The listing builds one solid part. Answer for the finished solid, in the listing's coordinates (mm). Face numbers are marked on the shaded views. Coordinates: 2 decimals unless noted, no trailing zeros. Order: outer loops, then holes, each group sorted by start corner. A loop starts at its lowest first (then second) coordinate and runs counter-clockwise, first axis right, second up.
```python
from build123d import *

# Parameters (mm, degrees)
F1_DEPTH = 150
F2_DEPTH = 25
F2_TAPER = -10


with BuildPart() as f1:
    # F0 (on Front) → F1 (new body)
    with BuildSketch(Plane.XZ):
        Polygon((47.8535592556, -25.4356767982), (42.105384171, -21.1245436221), (27.7349483222, -28.3097643405), (39.5187065005, -34.9201671779), (28.5936295986, -43.255019933), (45.6024929881, -43.255019933), (49.4760833681, -35.1725630462), (39.5187065005, -27.3510906845), align=None)
    extrude(amount=F1_DEPTH)

    # F1_face (on face) → F2 (join)
    with BuildSketch(Plane(origin=(39.6376889247, 0, -33.4798158905), x_dir=(1, 0, 0), z_dir=(0, 1, 0))):
        Polygon((2.4676952463, -12.3552722683), (8.2158703309, -8.0441390922), (-0.1189824242, -6.1287252059), (9.8383944433, 1.6927471558), (5.9648040634, 9.7752040425), (-11.0440593261, 9.7752040425), (-0.1189824242, 1.4403512875), (-11.9027406026, -5.1700515499), align=None)
    extrude(amount=F2_DEPTH, taper=F2_TAPER)


solid = f1.part
```
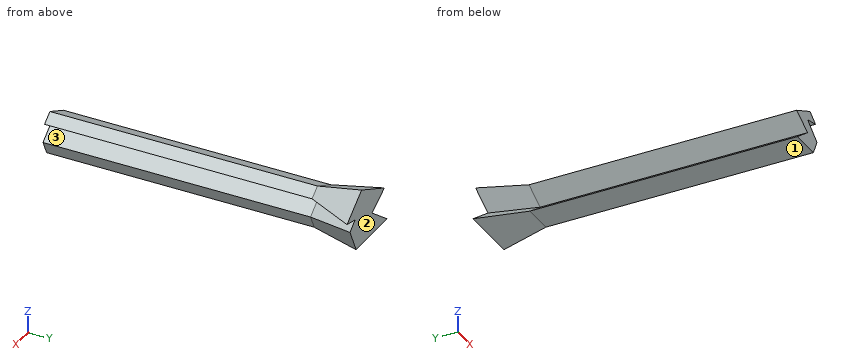
(1) Find section A-A (y = -104). Write down the section's boundary in (x, z).
(2) The mould has two halves that part along Z. Classify the marked faces 1, 2 and 3: released by +Z, released by -Z, zero draft, split by the parting line, or undercut.
(3) Each of these flat-tipped pins is pushed along its axis until it touches: pin 1 Ø8.5 at (x, y) = (37, -81) entering from -Z (3 decimals); pin 2 Ø2 at (y, z) = (-93, -30) entering from +X; pin 3 Ø5 at (y, z) = (-29.5, -31) entering from -X. Where does it stop, or does it pass through?
(4) Consider line 1 (Z direction, x = 37, y = -138); line 2 (Z direction, x = 47, y = -94.5); line 3 (X direction, y = 18.5, z = -32.5). Determine where each line is inside the solid, lowest interval first.
Findings below:
1. outline: (27.73, -28.31) - (39.52, -34.92) - (28.59, -43.26) - (45.6, -43.26) - (49.48, -35.17) - (39.52, -27.35) - (47.85, -25.44) - (42.11, -21.12) - close
2. face 1: released by -Z
2. face 2: zero draft
2. face 3: undercut
3. pin 1: stops at z = -43.255
3. pin 2: stops at x = 44.16
3. pin 3: stops at x = 28.07
4. line 1: z = -43.26 to -36.84, -33.51 to -23.68
4. line 2: z = -40.34 to -33.23, -25.63 to -24.8
4. line 3: x = 28.54 to 51.35
